```python
from build123d import *

# Parameters (mm, degrees)
F1_DEPTH = 4
F2_DEPTH = 8


with BuildPart() as f1:
    # F0 (on Top) → F1 (new body)
    with BuildSketch(Plane.XY):
        with BuildLine():
            ThreePointArc((-12.5, 0), (-8.838835, -8.838835), (0, -12.5))
            Line((0, -12.5), (0, -3.15))
            ThreePointArc((0, -3.15), (-2.227386, -2.227386), (-3.15, 0))
            Line((-3.15, 0), (-12.5, 0))
        make_face()
        with BuildLine():
            Line((0, 3.15), (0, 12.5))
            ThreePointArc((0, 12.5), (-8.838835, 8.838835), (-12.5, 0))
            Line((-12.5, 0), (-3.15, 0))
            ThreePointArc((-3.15, 0), (-2.227386, 2.227386), (0, 3.15))
        make_face()
        with BuildLine():
            Line((3.15, 0), (12.5, 0))
            ThreePointArc((12.5, 0), (8.838835, 8.838835), (0, 12.5))
            Line((0, 12.5), (0, 3.15))
            ThreePointArc((0, 3.15), (2.227386, 2.227386), (3.15, 0))
        make_face()
        with BuildLine():
            ThreePointArc((0, -12.5), (8.838835, -8.838835), (12.5, 0))
            Line((12.5, 0), (3.15, 0))
            ThreePointArc((3.15, 0), (2.227386, -2.227386), (0, -3.15))
            Line((0, -3.15), (0, -12.5))
        make_face()
    extrude(amount=F1_DEPTH)

    # F0 (on Top) → F2 (join)
    with BuildSketch(Plane.XY):
        with BuildLine():
            Line((3.15, 0), (12.5, 0))
            ThreePointArc((12.5, 0), (8.838835, 8.838835), (0, 12.5))
            Line((0, 12.5), (0, 3.15))
            ThreePointArc((0, 3.15), (2.227386, 2.227386), (3.15, 0))
        make_face()
        with BuildLine():
            ThreePointArc((-12.5, 0), (-8.838835, -8.838835), (0, -12.5))
            Line((0, -12.5), (0, -3.15))
            ThreePointArc((0, -3.15), (-2.227386, -2.227386), (-3.15, 0))
            Line((-3.15, 0), (-12.5, 0))
        make_face()
    extrude(amount=F2_DEPTH)


solid = f1.part
```
Can you work these out from the model? Positions are in its coordinate system, mm. A direction names the side the tool comes from. Give positions to 0.01 mm unless a question says otherwise; leave off trailing zeros. Loops run counter-clockwise (first coordinate to the right, second up) from the corner with the lowest first, then second, coordinate; pieces in that order, holes last. Notation, with made-up numbers: M -16.5,-28 L -11.5,-28 A18 cw -11.5,-20 Z; hole C -16,-30.5 d6. An arc over 180 degrees is marked long. One line per question, with ' | ' between items. Start each with the question number.
Q1. For pin 1 Ø4.5 at (y, z) = (-6, 6.5) entering from +X; pin 2 Ø1.5 at (x, y) = (-9.5, 7.5) entering from +Z; pin 3 Ø2 at (x, z) = (5.5, 3.5) entering from -Y, each with a flat end and sliding along its axis, tell me the tip position at first contact or that it passes through.
Q2. If we section it at A-A (z = 6): Please give me the cut outline in (x, y).
Q3. If we section it at B-B (z = 3.25): Please give me the cut outline in (x, y), plus the area to 3 significant figures.
Q4. If we section it at C-C (x = -0.75): Please give me the cut outline in (y, z).
Q5. If I drill on line 1 (Z direction, x = 6.25, y = -3); line 2 (Y direction, x = 2.25, z = 3.5), over which ranges is the centre line in solid material (lowest first)? Write a range as from..to.
Q6. For faces 1 (the flat face through (-6, 6, 4)), 2 (the flat face through (-6, -6, 8)), 3 (the flat face through (0, -8, 6)), which set-ups out of +Z, -Z, +X, -X, +Y, -Y let a thin tool reach every point of the face, with its end or its side?
Q7. If we section it at D-D (y = 7.5): Please give me the cut outline in (x, z), plus the area to 3 significant figures.
Computed:
1) pin 1: stops at x = 0 | pin 2: stops at z = 4 | pin 3: stops at y = -11.66
2) outline: M -12.5,0 A12.5 ccw 0,-12.5 L 0,-3.15 A3.15 cw -3.15,0 Z; M 0,3.15 A3.15 cw 3.15,0 L 12.5,0 A12.5 ccw 0,12.5 Z
3) outline: M -12.5,0 A12.5 ccw 0,-12.5 A12.5 ccw 12.5,0 A12.5 ccw 0,12.5 A12.5 ccw Z; hole M -3.15,0 A3.15 ccw 0,-3.15 A3.15 ccw 3.15,0 A3.15 ccw 0,3.15 A3.15 ccw Z | area: 460 mm²
4) outline: M -12.48,0 L -3.06,0 L -3.06,8 L -12.48,8 Z; M 3.06,0 L 12.48,0 L 12.48,4 L 3.06,4 Z
5) line 1: z = 0..4 | line 2: y = -12.3..-2.2, 2.2..12.3
6) face 1: +Z, -X, +Y | face 2: +Z, +X, -X, +Y, -Y | face 3: +Z, +X, -Y
7) outline: M -10,0 L 10,0 L 10,8 L 0,8 L 0,4 L -10,4 Z | area: 120 mm²
